Part model, mm, in its own coordinate system. Round coordinates to 2 decimals unless told otherwise and drop trailing zeros. Loops run counter-clockwise (first coordinate to the right, second up) from the corner with the lowest first, then second, coordinate; pieces in that order, holes last. Notation, with made-up numbers: M 16,1.25 L 61,1.25 A35 ccw 61,39.25 Z; hole C 41,25.25 d8. An arc over 180 degrees is marked long. Put each result on its own line as item: value. Start each with the question number.
1) Slice it at B-B on x = 55. Give the cut face in (y, z), then the cut area to 3 significant figures.
2) Drop flat-ended pins along their axis: pin 1 Ø3 at (y, z) = (-63.5, 2.5) entering from +X; pin 2 Ø3 at (x, z) = (60, 2) entering from -Y; pin 3 Ø3 at (x, z) = (63.5, 2) entering from +Y. Give the stop position or say it passes through.
3) Probe line 1 along Y through (x, z) = (5.5, 0.45); line 2 along Y through (x, z) = (0, 0.1); line 3 along X through (y, z) = (60, 0.35). List the from-to ranges inside material, lowest first.
4) Slice it at C-C on y = -50.5. Give the cut face in (x, z).
5) Slice it at A-A on z = 4.35. Give the cut face in (x, y), then the cut area to 4 significant figures.
```python
from build123d import *

# Parameters (mm, degrees)
F1_DEPTH = 0.5
F2_R     = 1
F3_DEPTH = 0.5
F4_W     = 15
F4_H     = 15
F5_DEPTH = 5


with BuildPart() as f1:
    # F0 (on Top) → F1 (new body)
    with BuildSketch(Plane.XY):
        Polygon((7.5, 67.5), (0, 67.5), (-7.5, 67.5), (-7.5, 52.5), (-1, 52.5), (-1, 7.5), (-7.5, 7.5), (-7.5, 1), (-52.5, 1), (-52.5, 7.5), (-67.5, 7.5), (-67.5, 0), (-67.5, -7.5), (-52.5, -7.5), (-52.5, -1), (-7.5, -1), (-7.5, -7.5), (-1, -7.5), (-1, -52.5), (-7.5, -52.5), (-7.5, -67.5), (0, -67.5), (7.5, -67.5), (7.5, -52.5), (1, -52.5), (1, -7.5), (7.5, -7.5), (7.5, -1), (52.5, -1), (52.5, -7.5), (67.5, -7.5), (67.5, 0), (67.5, 7.5), (52.5, 7.5), (52.5, 1), (7.5, 1), (7.5, 7.5), (1, 7.5), (1, 52.5), (7.5, 52.5), align=None)
    extrude(amount=F1_DEPTH)

    # F2 (on face) → F3 (cut, through all)
    with BuildSketch(Plane(origin=(0, 0, 0), x_dir=(1, 0, 0), z_dir=(0, 0, -1))):
        with Locations((0, -60)):
            Circle(F2_R)
    extrude(amount=-F3_DEPTH, mode=Mode.SUBTRACT)

    # F4 (on face) → F5 (join)
    with BuildSketch(Plane.XY.offset(0.5)):
        with Locations((-60, 0)):
            Rectangle(F4_W, F4_H)
        with Locations((0, 60)):
            Rectangle(F4_W, F4_H)
        with Locations((60, 0)):
            Rectangle(F4_W, F4_H)
        Rectangle(F4_W, F4_H)
        with Locations((0, -60)):
            Rectangle(F4_W, F4_H)
    extrude(amount=F5_DEPTH)


solid = f1.part
```
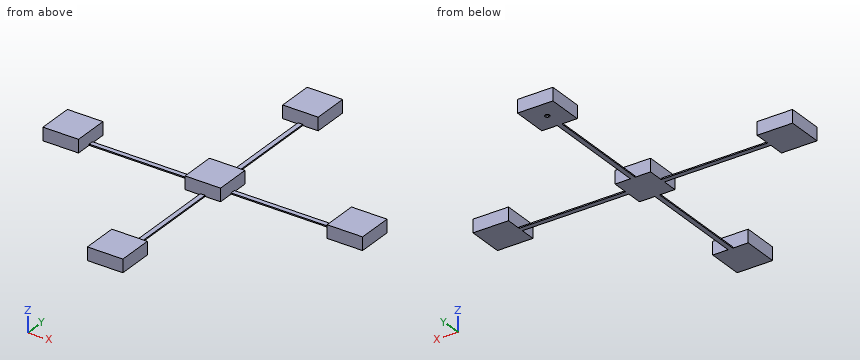
Recorded:
1. outline: M -7.5,0 L 7.5,0 L 7.5,5.5 L -7.5,5.5 Z
1. area: 82.5 mm2
2. pin 1: stops at x = 7.5
2. pin 2: stops at y = -7.5
2. pin 3: stops at y = 7.5
3. line 1: y = -67.5 to -52.5, -7.5 to 7.5, 52.5 to 67.5
3. line 2: y = -67.5 to 59, 61 to 67.5
3. line 3: x = -7.5 to -1, 1 to 7.5
4. outline: M -1,0 L 1,0 L 1,0.5 L -1,0.5 Z
5. outline: M -67.5,-7.5 L -52.5,-7.5 L -52.5,7.5 L -67.5,7.5 Z; M -7.5,-67.5 L 7.5,-67.5 L 7.5,-52.5 L -7.5,-52.5 Z; M -7.5,-7.5 L 7.5,-7.5 L 7.5,7.5 L -7.5,7.5 Z; M -7.5,52.5 L 7.5,52.5 L 7.5,67.5 L -7.5,67.5 Z; M 52.5,-7.5 L 67.5,-7.5 L 67.5,7.5 L 52.5,7.5 Z
5. area: 1,125 mm2
